CAD build for the part. Positions are in the model's coordinates, mm. A direction names the side the tool comes from. Round coordinates to 2 decimals unless told otherwise and drop trailing zeros. Write each loop counter-clockwise with the first axis right and the second up, starting at its lowest first coordinate (ties: lowest second). Pieces come first, ordered by that corner, then holes. Notation, with made-up numbers: (57.5, -24.5) - (101.5, -24.5) arc R18 ccw to (101.5, 1.5) - close; hole circle Ø2 at (20.5, -7). An arc over 180 degrees is marked (long way). Use one line per item in the form item = value. Start each with the question number.
Item 1: Drill centre lines: L1, parallel to Z at x = 0, y = -12.9 (3 decimals); L2, parallel to Y at x = 0.5, z = -6 (3 decimals); L3, parallel to X at y = -16.5, z = 3.5. Where is each one in solid material? Low to high.
Item 2: Pin check, flat tips, straight feed: pin 1 (10 mm diameter, centred on x = 2.5, z = -2.5, fed in from +Y); pin 2 (4 mm diameter, centred on y = -9, z = -2.5, fed in from -X); pin 3 (5 mm diameter, centred on x = -7.5, y = -12.5, fed in from -Z). Stop position of each tip, or through.
Item 3: Band-saw the part on A-A, the plane x = -0.5. List the corners of the cut face in (y, z) (3 decimals), and give its area (3 significant figures).
Item 4: Band-saw the part on B-B, the plane y = -9.75. List the corners of the cut face in (x, z) (3 decimals), and give its area (3 significant figures).
Item 5: Pull direction Z, two halves, no side cores. Call faces 1 (the flat face through (6.2, -25.4, 2.3)), 2 (the cylindrical face through (-1.294, -13.454, -5.827)), 3 (the cylindrical face through (-7.559, -12.522, -5.796)): +Z half, -Z half, draft (parallel to the pull), parting line (faces both ways), or undercut.
Item 6: Band-saw the part on C-C, the plane z = -4.5. List the corners of the cut face in (x, y) (3 decimals), and give its area (3 significant figures).
Item 7: Tool access for faces 4 (the flat face through (-0.1, 0, -6.2)), 5 (the flat face through (-5, -11.1, 5)), 6 (the flat face through (-5.5, -20.7, -3.12)): list every direction of +Z, -Z, +X, -X, +Y, -Y with a clear straight run to the whole face (end or side of a thin tool).
from build123d import *

# Parameters (mm, degrees)
F0_R     = 9.525
F1_DEPTH = 25.4
F3_R     = 5.969
F4_DEPTH = 25.401
F2_W     = 11.938
F2_H     = 11.938
F5_DEPTH = 11.0998
F7_DEPTH = 9.525


with BuildPart() as f1:
    # F0 (on Front) → F1 (new body)
    with BuildSketch(Plane.XZ):
        Circle(F0_R)
    extrude(amount=F1_DEPTH)

    # F3 (on Front) → F4 (cut, through all)
    with BuildSketch(Plane.XZ):
        Circle(F3_R)
    extrude(amount=F4_DEPTH, mode=Mode.SUBTRACT)

    # F2 (on Front) → F5 (cut)
    with BuildSketch(Plane.XZ):
        Rectangle(F2_W, F2_H)
    extrude(amount=F5_DEPTH, mode=Mode.SUBTRACT)

    # F6 (on face) → F7 (cut)
    with BuildSketch(Plane.XZ.offset(25.4)):
        Polygon((3.65125, 6.324151), (-3.65125, 6.324151), (-7.3025, 0), (-3.65125, -6.324151), (3.65125, -6.324151), (7.3025, 0), align=None)
    extrude(amount=-F7_DEPTH, mode=Mode.SUBTRACT)


solid = f1.part
Determined:
q1.L1 = -9.525 to -5.969, 5.969 to 9.525
q1.L2 = -15.875 to 0
q1.L3 = -8.86 to -5.28, 5.28 to 8.86
q2.pin_1 = 0
q2.pin_2 = -9.51
q2.pin_3 = -8.11
q3.outline = (-25.4, -9.512) - (0, -9.512) - (0, -5.969) - (-11.1, -5.969) - (-11.1, -5.948) - (-15.875, -5.948) - (-15.875, -6.324) - (-25.4, -6.324) - close; (-25.4, 6.324) - (-15.875, 6.324) - (-15.875, 5.948) - (-11.1, 5.948) - (-11.1, 5.969) - (0, 5.969) - (0, 9.512) - (-25.4, 9.512) - close
q3.area = 173 mm²
q4.outline = circle Ø19.05 at (0, 0); hole (-5.969, -5.969) - (5.969, -5.969) - (5.969, 5.969) - (-5.969, 5.969) - close
q4.area = 143 mm²
q5.face_1 = draft
q5.face_2 = undercut
q5.face_3 = parting line
q6.outline = (-8.395, -25.4) - (-4.704, -25.4) - (-4.704, -15.875) - (-3.922, -15.875) - (-3.922, -11.1) - (-5.969, -11.1) - (-5.969, 0) - (-8.395, 0) - close; (3.922, -15.875) - (4.704, -15.875) - (4.704, -25.4) - (8.395, -25.4) - (8.395, 0) - (5.969, 0) - (5.969, -11.1) - (3.922, -11.1) - close
q6.area = 167 mm²
q7.face_4 = +Z, -Z, +X, -X, +Y
q7.face_5 = +Y
q7.face_6 = -Y
